Could you check a few things on this model? Use its own coordinates, in mm. A direction names the side the tool comes from. Round coordinates to 2 decimals unless told otherwise and drop trailing zeros. Loops run counter-clockwise (first coordinate to the right, second up) from the corner with the lowest first, then second, coordinate; pieces in that order, holes last.
from build123d import *

# Parameters (mm, degrees)
ESBO_O1_R                = 4.5
RESSALTO_EXTRUS_O1_DEPTH = 5
ESBO_O3_R                = 0.9
CORTE_EXTRUS_O4_DEPTH    = 11.8
ESBO_O5_W                = 1.8
ESBO_O5_H                = 6.8
CORTE_EXTRUS_O5_DEPTH    = 1


with BuildPart() as part:
    # Esboço1 → Ressalto-extrusão1 (new body)
    with BuildSketch(Plane.XY):
        with BuildLine():
            Line((7.237292739, 13.882644275), (4.931205446, 10.964033635))
            ThreePointArc((4.931205446, 10.964033635), (3.383365404, 11.536015744), (1.77178072, 11.89065237))
            Line((1.77178072, 11.89065237), (1.451023847, 15.579942687))
            ThreePointArc((1.451023847, 15.579942687), (1.141313879, 16.220426504), (0.484122849, 16.4928962))
            ThreePointArc((0.484122849, 16.4928962), (0.017522037, 16.499990696), (-0.449092791, 16.493887221))
            ThreePointArc((-0.449092791, 16.493887221), (-1.103704511, 16.225768855), (-1.417126065, 15.591599404))
            Line((-1.417126065, 15.591599404), (-1.779210104, 11.889542973))
            ThreePointArc((-1.779210104, 11.889542973), (-3.390572883, 11.533899437), (-4.938055227, 10.960950291))
            Line((-4.938055227, 10.960950291), (-7.202474013, 13.891164545))
            ThreePointArc((-7.202474013, 13.891164545), (-7.809290312, 14.262531969), (-8.509462826, 14.136443768))
            ThreePointArc((-8.509462826, 14.136443768), (-8.905827982, 13.890148593), (-9.295069567, 13.632743002))
            ThreePointArc((-9.295069567, 13.632743002), (-9.700808257, 13.053277663), (-9.621617356, 12.350331887))
            Line((-9.621617356, 12.350331887), (-7.924739018, 9.040206424))
            ThreePointArc((-7.924739018, 9.040206424), (-9.088028236, 7.869851554), (-10.08009353, 6.55122394))
            Line((-10.08009353, 6.55122394), (-13.569237263, 7.792039811))
            ThreePointArc((-13.569237263, 7.792039811), (-14.280500006, 7.776384308), (-14.80135418, 7.291770323))
            ThreePointArc((-14.80135418, 7.291770323), (-15.001640543, 6.870282455), (-15.189927432, 6.443299203))
            ThreePointArc((-15.189927432, 6.443299203), (-15.217973923, 5.736463043), (-14.771313119, 5.187921259))
            Line((-14.771313119, 5.187921259), (-11.554219287, 3.320668211))
            ThreePointArc((-11.554219287, 3.320668211), (-11.900098837, 1.707181407), (-12.02177336, 0.061530278))
            Line((-12.02177336, 0.061530278), (-15.627863558, -0.781002507))
            ThreePointArc((-15.627863558, -0.781002507), (-16.21775185, -1.178710425), (-16.393920163, -1.867988679))
            ThreePointArc((-16.393920163, -1.867988679), (-16.334538228, -2.330849819), (-16.262090664, -2.791846566))
            ThreePointArc((-16.262090664, -2.791846566), (-15.903540395, -3.401638061), (-15.231221337, -3.621617713))
            Line((-15.231221337, -3.621617713), (-11.51531657, -3.453158696))
            ThreePointArc((-11.51531657, -3.453158696), (-10.93397214, -4.997506773), (-10.14662509, -6.447698813))
            Line((-10.14662509, -6.447698813), (-12.724753595, -9.106082048))
            ThreePointArc((-12.724753595, -9.106082048), (-13.005982071, -9.759572927), (-12.781532328, -10.434674473))
            ThreePointArc((-12.781532328, -10.434674473), (-12.48133544, -10.791953745), (-12.171155012, -11.140600777))
            ThreePointArc((-12.171155012, -11.140600777), (-11.53984516, -11.459743115), (-10.855324398, -11.28131865))
            Line((-10.855324398, -11.28131865), (-7.820382206, -9.130632116))
            ThreePointArc((-7.820382206, -9.130632116), (-6.496386543, -10.115521864), (-5.049995046, -10.909829088))
            Line((-5.049995046, -10.909829088), (-5.781624274, -14.540044879))
            ThreePointArc((-5.781624274, -14.540044879), (-5.664904879, -15.241839982), (-5.111098288, -15.68842485))
            ThreePointArc((-5.111098288, -15.68842485), (-4.665396838, -15.826688609), (-4.215963642, -15.952292956))
            ThreePointArc((-4.215963642, -15.952292956), (-3.512330623, -15.879460702), (-3.032938663, -15.359280625))
            Line((-3.032938663, -15.359280625), (-1.642531748, -11.909194354))
            ThreePointArc((-1.642531748, -11.909194354), (0.003755879, -12.021930236), (1.649972743, -11.908165713))
            Line((1.649972743, -11.908165713), (2.997129903, -15.357646195))
            ThreePointArc((2.997129903, -15.357646195), (3.474739585, -15.884930537), (4.182073344, -15.961211187))
            ThreePointArc((4.182073344, -15.961211187), (4.631772295, -15.836561666), (5.077766396, -15.699244836))
            ThreePointArc((5.077766396, -15.699244836), (5.630324069, -15.257561714), (5.752383667, -14.560779526))
            Line((5.752383667, -14.560779526), (5.056810935, -10.90667153))
            ThreePointArc((5.056810935, -10.90667153), (6.502705837, -10.111460701), (7.826085845, -9.125743863))
            Line((7.826085845, -9.125743863), (10.824316513, -11.299303357))
            ThreePointArc((10.824316513, -11.299303357), (11.511178782, -11.484667883), (12.147466239, -11.166425748))
            ThreePointArc((12.147466239, -11.166425748), (12.458386452, -10.81843829), (12.759341481, -10.461797406))
            ThreePointArc((12.759341481, -10.461797406), (12.985390652, -9.791494687), (12.711364828, -9.139333809))
            Line((12.711364828, -9.139333809), (10.150651876, -6.441357558))
            ThreePointArc((10.150651876, -6.441357558), (10.937092637, -4.990673837), (11.517471987, -3.445962816))
            Line((11.517471987, -3.445962816), (15.21485911, -3.65351154))
            ThreePointArc((15.21485911, -3.65351154), (15.89290005, -3.438104324), (16.256124433, -2.826379032))
            ThreePointArc((16.256124433, -2.826379032), (16.329550936, -2.365537195), (16.389915799, -1.902803219))
            ThreePointArc((16.389915799, -1.902803219), (16.217687452, -1.21669728), (15.63457747, -0.816214183))
            Line((15.63457747, -0.816214183), (12.021732567, 0.069041925))
            ThreePointArc((12.021732567, 0.069041925), (11.899029803, 1.714616707), (11.552142152, 3.327887077))
            Line((11.552142152, 3.327887077), (14.774791444, 5.152244377))
            ThreePointArc((14.774791444, 5.152244377), (15.228737846, 5.700033066), (15.203577979, 6.411023056))
            ThreePointArc((15.203577979, 6.411023056), (15.016198378, 6.838405244), (14.816807657, 7.260317546))
            ThreePointArc((14.816807657, 7.260317546), (14.300983076, 7.744392916), (13.593922234, 7.766047679))
            Line((13.593922234, 7.766047679), (10.07599811, 6.557521086))
            ThreePointArc((10.07599811, 6.557521086), (9.083109081, 7.875528562), (7.919088807, 9.045156337))
            Line((7.919088807, 9.045156337), (9.643831887, 12.322199108))
            ThreePointArc((9.643831887, 12.322199108), (9.729558977, 13.028450232), (9.324002941, 13.612970622))
            ThreePointArc((9.324002941, 13.612970622), (8.935308934, 13.871202336), (8.539467774, 14.118338788))
            ThreePointArc((8.539467774, 14.118338788), (7.843817619, 14.246693081), (7.237292739, 13.882644275))
        make_face()
        Circle(ESBO_O1_R, mode=Mode.SUBTRACT)
    extrude(amount=RESSALTO_EXTRUS_O1_DEPTH)

    # Esboço3 → Corte-extrusão4 (cut)
    with BuildSketch(Plane(origin=(0, 0, 0), x_dir=(-1, 0, 0), z_dir=(0, 0, -1))):
        with Locations((3.4, 7.28)):
            Circle(ESBO_O3_R)
        with Locations((0, 7.28)):
            Circle(ESBO_O3_R)
        with Locations((-3.4, 7.28)):
            Circle(ESBO_O3_R)
        with Locations((7.28, -3.4)):
            Circle(ESBO_O3_R)
        with Locations((7.28, 0)):
            Circle(ESBO_O3_R)
        with Locations((7.28, 3.4)):
            Circle(ESBO_O3_R)
        with Locations((-3.4, -7.28)):
            Circle(ESBO_O3_R)
        with Locations((0, -7.28)):
            Circle(ESBO_O3_R)
        with Locations((3.4, -7.28)):
            Circle(ESBO_O3_R)
        with Locations((-7.28, 3.4)):
            Circle(ESBO_O3_R)
        with Locations((-7.28, 0)):
            Circle(ESBO_O3_R)
        with Locations((-7.28, -3.4)):
            Circle(ESBO_O3_R)
    extrude(amount=-CORTE_EXTRUS_O4_DEPTH, mode=Mode.SUBTRACT)

    # Esboço5 → Corte-extrusão5 (cut)
    with BuildSketch(Plane(origin=(0, 0, 0), x_dir=(-1, 0, 0), z_dir=(0, 0, -1))):
        with Locations((7.28, 0)):
            Rectangle(ESBO_O5_W, ESBO_O5_H)
        with Locations((-7.28, 0)):
            Rectangle(ESBO_O5_W, ESBO_O5_H)
    extrude(amount=-CORTE_EXTRUS_O5_DEPTH, mode=Mode.SUBTRACT)


solid = part.part
Item 1: If I drill on line 1 along Y through (x, z) = (8, 1.4); line 2 along Y through (x, z) = (-4, 4.65); line 3 along Y through (x, z) = (-3.4, 1.85), over which ranges is the centre line in solid material (lowest first)?
Results list:
line 1: y = -9.25 to -3.94, -2.86 to -0.54, 0.54 to 2.86, 3.94 to 8.97, 9.2 to 14.26
line 2: y = -15.98 to -7.95, -6.61 to -2.06, 2.06 to 6.61, 7.95 to 11.34
line 3: y = -15.81 to -8.18, -6.38 to -2.95, 2.95 to 6.38, 8.18 to 11.53
Item 2: If we section it at D-D, the plane z = 3.7: Count the separate pieces of the cut face and the enclosed holes in it, then the cut area to 3 significant figures.
Results list:
separate pieces: 1
enclosed holes: 13
area: 511 mm2
Item 3: For faces 1 (the flat face through (-1.596, 13.766, 2.465)), 2 (the flat face through (8.77, 10.66, 2.46)), 3 (the flat face through (7, -2, 1)), which set-ups out of +Z, -Z, +X, -X, +Y, -Y let a thin tool reach every point of the face, with its end or its side?
Results list:
face 1: +Z, -Z, +Y
face 2: +Z, -Z, +X
face 3: -Z
Item 4: If we section it at B-B, the plane y = -14: Please give me the cut outline in (x, z), then the cut area to 3 significant figures.
Results list:
outline: (-5.67, 0) - (-2.49, 0) - (-2.49, 5) - (-5.67, 5) - close; (2.47, 0) - (5.65, 0) - (5.65, 5) - (2.47, 5) - close
area: 31.8 mm2
Item 5: Will these pins go through, and if not, where does the flat tip stop? pin 1 (1.4 mm diameter, centred on x = 7.28, y = -3.4, fed in from -Z); pin 2 (1 mm diameter, centred on y = -4.5, z = 0.5, fed in from -X); pin 3 (0.5 mm diameter, centred on x = -7, y = 1.5, fed in from -Z); pin 4 (1 mm diameter, centred on y = -8, z = 2.5, fed in from -X).
Results list:
pin 1: passes through
pin 2: stops at x = -11.34
pin 3: stops at z = 1
pin 4: stops at x = -12.14
Item 6: If we section it at A-A, the plane x = 0: Please give me the cut outline in (y, z), then the cut area to 3 significant figures.
Results list:
outline: (-12.02, 0) - (-8.18, 0) - (-8.18, 5) - (-12.02, 5) - close; (-6.38, 0) - (-4.5, 0) - (-4.5, 5) - (-6.38, 5) - close; (4.5, 0) - (6.38, 0) - (6.38, 5) - (4.5, 5) - close; (8.18, 0) - (16.5, 0) - (16.5, 5) - (8.18, 5) - close
area: 79.6 mm2
Item 7: If we section it at C-C, the plane y = 11.5: Please give me the cut outline in (x, z), then the cut area to 3 significant figures.
Results list:
outline: (-9.19, 0) - (-5.35, 0) - (-5.35, 5) - (-9.19, 5) - close; (-3.5, 0) - (3.5, 0) - (3.5, 5) - (-3.5, 5) - close; (5.35, 0) - (9.21, 0) - (9.21, 5) - (5.35, 5) - close
area: 73.5 mm2
Item 8: We'd pull the mould along Y, two halves only. Please class faces 4 (the flat face through (1.614, 13.709, 2.465)), 5 (the cylindrical face through (-0.02, -12.02, 2.46)), 6 (the cylindrical face through (-10.94, -4.98, 2.46)): released by +Y, released by -Y, zero draft, split by the parting line, or undercut.
Results list:
face 4: released by +Y
face 5: released by -Y
face 6: undercut
